Geometry check sheet. Reference: drawing and pictorial views, mm from the part's lowest x, y, z. Round coordinates to 2 decimals unless told otherwise and drop trailing zeros. Write each loop counter-clockwise with the first axis right and the second up, starting at its lowest first coordinate (ties: lowest second). Pieces come first, ordered by that corner, then holes. Notation, with made-up numbers: M 70.25,21.25 L 98.25,21.25 A17 cw 98.25,52.25 Z; hole C 8,-1.5 d5. An arc over 180 degrees is marked long. One line per question, with ' | ' between items.
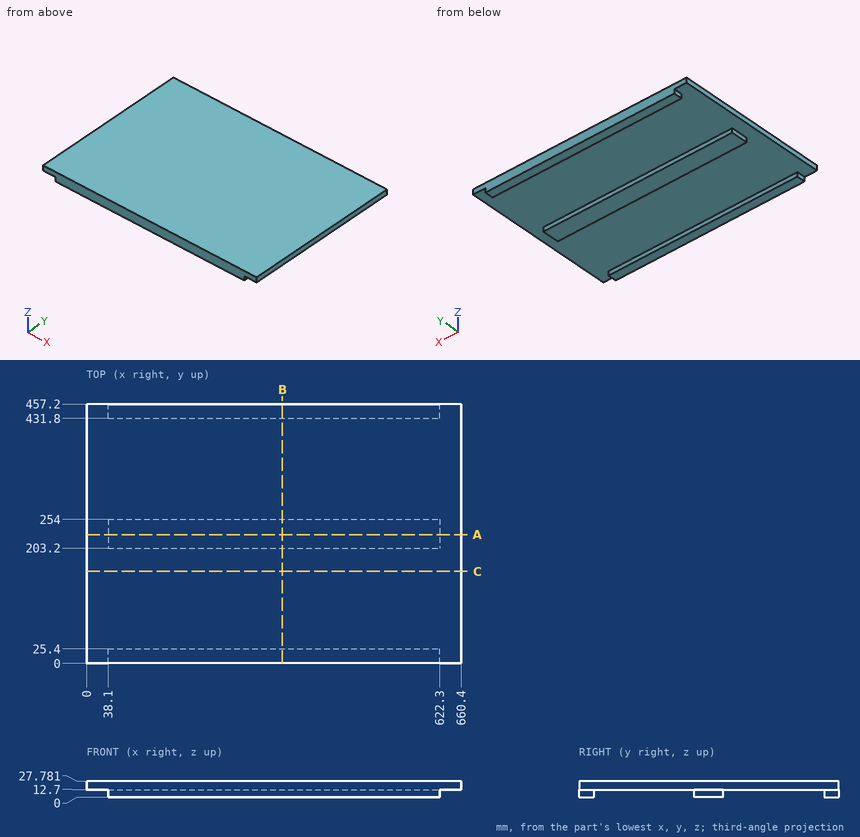
1. Section check B-B, the plane x = 345.5. Record the cut outline in (y, z).
Results:
outline: M 0,0 L 25.4,0 L 25.4,12.7 L 203.2,12.7 L 203.2,0 L 254,0 L 254,12.7 L 431.8,12.7 L 431.8,0 L 457.2,0 L 457.2,27.78 L 0,27.78 Z
2. Section check C-C, the plane y = 162. Record the cut outline in (x, z).
Results:
outline: M 0,12.7 L 660.4,12.7 L 660.4,27.78 L 0,27.78 Z
3. Go/stop test with flat-tipped pins: P1, Ø10, axis at y = 445.5, z = 5.5, coming from the +X side; P2, Ø8, axis at x = 395, y = 344, coming from the -Z side; P3, Ø4, axis at y = 18, z = 4, coming from the -X side. Record where each tip stops, or that it passes through.
Results:
P1: stops at x = 622.3 | P2: stops at z = 12.7 | P3: stops at x = 38.1
4. Thickness scan on line 1 (Y direction, x = 255, z = 4.75); line 2 (Z direction, x = 49, y = 399.5); line 3 (X direction, y = 253.5, z = 9.25). Record the ranges inside material, lowest first.
Results:
line 1: y = 0 to 25.4, 203.2 to 254, 431.8 to 457.2 | line 2: z = 12.7 to 27.78 | line 3: x = 38.1 to 622.3
5. Section check A-A, the plane y = 227. Record the cut outline in (x, z).
Results:
outline: M 0,12.7 L 38.1,12.7 L 38.1,0 L 622.3,0 L 622.3,12.7 L 660.4,12.7 L 660.4,27.78 L 0,27.78 Z
